from build123d import *

# Parameters (mm, degrees)
F0_R           = 41.15773508
F1_DEPTH       = 127
F2_R           = 13.8288894668
F3_DEPTH       = 139.7
F4_R           = 25.4
F5_DEPTH       = 127.0010001
F9_R           = 13.8288903
F10_DEPTH      = 71.12
F10_DEPTH_BACK = 25.4
F6_R           = 12.5475422144
F11_DEPTH      = 130.13189


with BuildPart() as f1:
    # F0 (on Front) → F1 (new body)
    with BuildSketch(Plane.XZ):
        Circle(F0_R)
    extrude(amount=-F1_DEPTH)

    # F2 (on Right) → F3 (join)
    with BuildSketch(Plane.YZ):
        with Locations((100.965000689, 0)):
            Circle(F2_R)
    extrude(amount=F3_DEPTH)

    # F4 (on face) → F5 (cut, through all)
    with BuildSketch(Plane.XZ):
        Circle(F4_R)
    extrude(amount=-F5_DEPTH, mode=Mode.SUBTRACT)

    # F9 (on line) → F10 (join, two sides)
    with BuildSketch(Plane(origin=(45.6729605794, 46.6137044132, 0), x_dir=(-0.7142777152, 0.6998623761, 0), z_dir=(0.6998623761, 0.7142777152, 0))) as f10_sk:
        Circle(F9_R)
    extrude(amount=F10_DEPTH)
    extrude(f10_sk.sketch, amount=-F10_DEPTH_BACK)

    # F6 (on face) → F11 (cut)
    with BuildSketch(Plane.YZ.offset(139.7)):
        with Locations((100.965000689, 0)):
            Circle(F6_R)
    extrude(amount=-F11_DEPTH, mode=Mode.SUBTRACT)


solid = f1.part
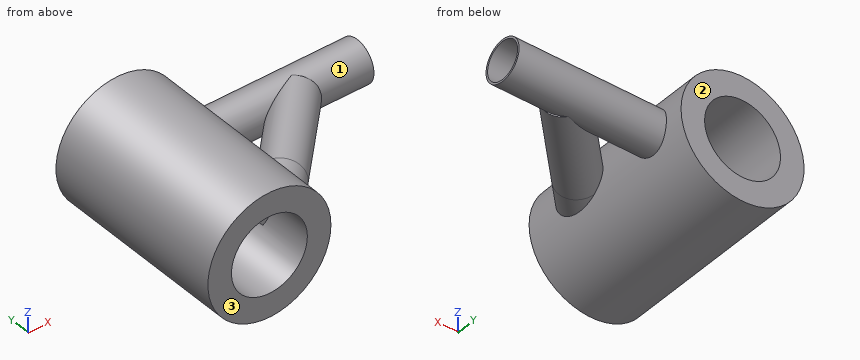
Part model, mm, in its own coordinate system. Face numbers are marked on the shaded views. Give positions to 0.01 mm unless a question says otherwise; leave off trailing zeros. Order: outer loops, then holes, each group sorted by start corner. A loop starts at its lowest first (then second) coordinate and runs counter-clockwise, first axis right, second up. Notation, with made-up numbers: (16.25, 19.25) - (66.25, 19.25) arc R12 cw to (66.25, 37.25) - close; hole circle Ø6 at (8, 14). An arc over 180 degrees is marked (long way). Use a Markdown table: item, result.
1) Saw through at A-A on x = 0. List the corners of the cut face in (y, z), plus the area to 3 significant figures.
Checked values:
| item | result |
|---|---|
| outline | (0, -41.16) - (127, -41.16) - (127, -25.4) - (0, -25.4) - close; (0, 25.4) - (127, 25.4) - (127, 41.16) - (0, 41.16) - close |
| area | 4,000 mm² |
2) Probe L1, parallel to Y at x = 117, z = -1; L2, parallel to Z at x = 0, y = 34; L3, parallel to Y at x = 74, z = 0. List the from-to ranges inside material, lowest first. Write a range as from..to.
Checked values:
| item | result |
|---|---|
| L1 | 87.17..88.46, 113.47..114.76 |
| L2 | -41.16..-25.4, 25.4..41.16 |
| L3 | 55.76..88.42, 113.51..114.79 |
3) Saw through at D-D on y = 106. List the corners of the cut face in (x, z).
Checked values:
| item | result |
|---|---|
| outline | (22.65, -11.49) arc R25.4 cw (long way) to (22.65, 11.49) - (139.7, 11.49) - (139.7, 12.88) - (39.09, 12.88) arc R41.16 ccw (long way) to (39.09, -12.88) - (139.7, -12.88) - (139.7, -11.49) - close |
4) Two-plate mould, pull along Y, no slides. Class the marked faces 1, 2 and 3: +Y half, -Y half, draft (parallel to the pull), parting line (faces both ways), or undercut.
Checked values:
| item | result |
|---|---|
| face 1 | undercut |
| face 2 | +Y half |
| face 3 | -Y half |
5) Saw through at B-B on y = 19. List the corners of the cut face in (x, z).
Checked values:
| item | result |
|---|---|
| outline | circle Ø82.32 at (0, 0); hole circle Ø50.8 at (0, 0) |
6) Flat gauge pins, fed straight in: P1, Ø4, axis at x = -13.5, y = 100.5, coming from the +Z side; P2, Ø4, axis at x = 62.5, y = 52.5, coming from the -Z side; P3, Ø2, axis at y = 54.5, z = -22, coming from the +X side. Where does each tip first touch, or does it go through?
Checked values:
| item | result |
|---|---|
| P1 | z = 39.52 |
| P2 | z = -12.51 |
| P3 | x = 35.4 |
7) Saw through at C-C on x = 34. List the corners of the cut face in (y, z) (3 decimals).
Checked values:
| item | result |
|---|---|
| outline | (0, -23.194) - (127, -23.194) - (127, 23.194) - (0, 23.194) - close; hole circle Ø25.095 at (100.965, 0) |
